from build123d import *

# Parameters (mm, degrees)
SKETCH1_R               = 1.75
BOSS_EXTRUDE1_DEPTH     = 1.5
BOSS_EXTRUDE2_START     = -72
BOSS_EXTRUDE2_DEPTH     = 72
BOSS_EXTRUDE4_DEPTH     = 2
SKETCH5_R               = 1.75
CUT_EXTRUDE1_DEPTH      = 2
CUT_EXTRUDE2_DEPTH      = 152.713437324
CUT_EXTRUDE2_DEPTH_BACK = 152.713437324
SKETCH6_W               = 72
SKETCH6_H               = 11.5
FILLET1_R               = 2
SKETCH8_W               = 36
SKETCH8_H               = 18
CUT_EXTRUDE3_DEPTH      = 22.4262221
SKETCH11_W              = 3
SKETCH11_H              = 15
BOSS_EXTRUDE7_DEPTH     = 15
CUT_EXTRUDE5_REACH      = 154.64
FILLET3_R               = 5


with BuildPart() as part:
    # Sketch1 → Boss-Extrude1 (new body)
    with BuildSketch(Plane.XY):
        with BuildLine():
            Line((-32.5, -138.9), (32.5, -138.9))
            Line((32.5, -138.9), (36, -138.9))
            Line((36, -138.9), (36, -136.815047169))
            ThreePointArc((36, -136.815047169), (37.65, -133.9), (36, -130.984952831))
            Line((36, -130.984952831), (36, -8.615047169))
            ThreePointArc((36, -8.615047169), (37.65, -5.7), (36, -2.784952831))
            Line((36, -2.784952831), (36, 0))
            Line((36, 0), (-36, 0))
            Line((-36, 0), (-36, -2.784952831))
            ThreePointArc((-36, -2.784952831), (-37.65, -5.7), (-36, -8.615047169))
            Line((-36, -8.615047169), (-36, -130.984952831))
            ThreePointArc((-36, -130.984952831), (-37.65, -133.9), (-36, -136.815047169))
            Line((-36, -136.815047169), (-36, -138.9))
            Line((-36, -138.9), (-32.5, -138.9))
        make_face()
        with Locations((-34.25, -133.9)):
            Circle(SKETCH1_R, mode=Mode.SUBTRACT)
        with Locations((34.25, -133.9)):
            Circle(SKETCH1_R, mode=Mode.SUBTRACT)
        with Locations((34.25, -5.7)):
            Circle(SKETCH1_R, mode=Mode.SUBTRACT)
        with Locations((-34.25, -5.7)):
            Circle(SKETCH1_R, mode=Mode.SUBTRACT)
    extrude(amount=BOSS_EXTRUDE1_DEPTH)

    # Sketch2 → Boss-Extrude2 (add)
    with BuildSketch(Plane.ZY.offset(36).offset(BOSS_EXTRUDE2_START)):
        Polygon((1.5, -141.1), (1.5, -138.9), (0, -138.9), (0, -139.1), (-40, -139.1), (-40, -141.1), align=None)
    extrude(amount=BOSS_EXTRUDE2_DEPTH)

    # Sketch4 → Boss-Extrude4 (add)
    with BuildSketch(Plane.XZ.offset(141.1)):
        with BuildLine():
            Line((-36, -15.904411924), (-36, -24.211404996))
            ThreePointArc((-36, -24.211404996), (-38.768391924, -20.05790846), (-36, -15.904411924))
        make_face()
        with BuildLine():
            Line((36, -15.879321263), (36, -24.236495657))
            ThreePointArc((36, -24.236495657), (38.8298476, -20.05790846), (36, -15.879321263))
        make_face()
    extrude(amount=-BOSS_EXTRUDE4_DEPTH)

    # Sketch5 → Cut-Extrude1 (cut)
    with BuildSketch(Plane.XZ.offset(141.1)):
        with Locations(Location((-34.25, -20, 0), (0, 0, 270))):
            Circle(SKETCH5_R)
        with Locations(Location((34.25, -20, 0), (0, 0, 270))):
            Circle(SKETCH5_R)
    extrude(amount=-CUT_EXTRUDE1_DEPTH, mode=Mode.SUBTRACT)

    # Sketch6 → Cut-Extrude2 (cut, two sides: drawn at the far end of the back side and taken through both)
    with BuildSketch(Plane.XZ.offset(141.1).offset(-CUT_EXTRUDE2_DEPTH_BACK)):
        with Locations((0, -34.25)):
            Rectangle(SKETCH6_W, SKETCH6_H)
    extrude(amount=CUT_EXTRUDE2_DEPTH + CUT_EXTRUDE2_DEPTH_BACK, mode=Mode.SUBTRACT)

    # Fillet1
    fillet1_edges = [part.edges().sort_by_distance(p)[0] for p in [
        (36, -140.1, -28.5),
        (-36, -140.1, -28.5),
    ]]
    fillet(fillet1_edges, radius=FILLET1_R)

    # Sketch8 → Cut-Extrude3 (cut)
    with BuildSketch(Plane.XZ.offset(141.1)):
        with Locations((-9, -14.5)):
            Rectangle(SKETCH8_W, SKETCH8_H)
    extrude(amount=-CUT_EXTRUDE3_DEPTH, mode=Mode.SUBTRACT)

    # Sketch11 → Boss-Extrude7 (add)
    with BuildSketch(Plane(origin=(0, -139.1, 0), x_dir=(1, 0, 0), z_dir=(0, 1, 0))):
        with Locations((10.5, 7.5)):
            Rectangle(SKETCH11_W, SKETCH11_H)
    extrude(amount=BOSS_EXTRUDE7_DEPTH)

    # Sketch12 → Cut-Extrude5 (cut, up to next)
    with BuildSketch(Plane(origin=(12, 0, 0), x_dir=(0, 0, -1), z_dir=(1, 0, 0)), mode=Mode.PRIVATE) as cut_extrude5_sk1:
        Polygon((0, -124.1), (15, -139.1), (15, -124.1), align=None)
    cut_extrude5_tool1 = extrude(cut_extrude5_sk1.sketch, amount=-CUT_EXTRUDE5_REACH, mode=Mode.PRIVATE) & part.part
    add(cut_extrude5_tool1.solids().sort_by_distance((12, -129.1, -10))[0], mode=Mode.SUBTRACT)

    # Fillet3
    fillet3_edges = [part.edges().sort_by_distance(p)[0] for p in [
        (36, -140.1, -24.236495657),
        (36, -140.1, -15.879321263),
        (-36, -140.1, -15.904411924),
        (-36, -140.1, -24.211404996),
    ]]
    fillet(fillet3_edges, radius=FILLET3_R)


solid = part.part
The listing builds one solid part. Answer for the finished solid, in the listing's coordinates (mm). A direction names the side the tool comes from. Round coordinates to 2 decimals unless told otherwise and drop trailing zeros. Write each loop counter-clockwise with the first axis right and the second up, starting at its lowest first coordinate (ties: lowest second). Pieces come first, ordered by that corner, then holes. Notation, with made-up numbers: (39.5, 50) - (55.5, 50) arc R22 cw to (55.5, 56) - close; hole circle Ø9 at (43.5, -12.5). An arc over 180 degrees is marked (long way). Use a Markdown table: item, result. Add a question column.
1. A tool of negligible diameter and unlimited length cuts with its end or side. For faces 1 (the face through (36, -140, -6)), 2 (the face through (9, -136, -6)), 3 (the face through (-36, -140, -6)), 4 (the face through (12, -133, -6)), from which of +Z, -Z, +X, -X, +Y, -Y can it reach the whole face along a straight path? Write none if from no direction.
2. Consider line 1 (Y direction, x = -34.25, z = 0.45); line 2 (X direction, y = -139.7, z = -20); line 3 (X direction, y = -133.9, z = 0.9). Determine where each line is inside the solid, lowest interval first.
3. Flat-ended cylindrical pins translate along their axes: P1, Ø7.5, axis at y = -131, z = -6, coming from the +X side; P2, Ø3.5, axis at y = -139.5, z = -7, coming from the -X side; P3, Ø4, axis at x = 28.5, y = -117, coming from the -Z side. Find the tip coordinate at first contact, or state that the pin passes through.
4. The part is cut by section B-B (x = -4). Write down the section's boundary in (y, z).
5. For a pull along Z with two mould halves and no side action, classify faces 5 (the face through (34.33, -140.11, -18.25)), 6 (the face through (10.5, -131.5, -7.4)), 7 (the face through (-34.63, -135.61, 0.74)), 8 (the face through (-34.17, -140.11, -18.25)) as +Z half, -Z half, draft (parallel to the pull), parting line (faces both ways), or undercut.
6. The part is cut by section A-A (z = -8.5). Write down the section's boundary in (x, y).
7. The part is cut by section D-D (z = -2.5). Write down the section's boundary in (x, y), and give its area (4 significant figures).
8. The part is cut by section C-C (y = -133.9). Write down the section's boundary in (x, z).
Reported:
| question | item | result |
|---|---|---|
| 1 | face 1 | +Z, +X, -Y |
| 1 | face 2 | +Y |
| 1 | face 3 | +Z, -X, -Y |
| 1 | face 4 | -Z, +X, +Y |
| 2 | line 1 | -141.1 to -135.65, -132.15 to -7.45, -3.95 to 0 |
| 2 | line 2 | -38.77 to -36, -32.5 to -27, 9 to 32.5, 36 to 38.83 |
| 2 | line 3 | -37.65 to -36, -32.5 to 32.5, 36 to 37.65 |
| 3 | P1 | x = 12 |
| 3 | P2 | x = -36 |
| 3 | P3 | z = 0 |
| 4 | outline | (-141.1, -28.5) - (-139.1, -28.5) - (-139.1, -23.5) - (-141.1, -23.5) - close; (-141.1, -5.5) - (-139.1, -5.5) - (-139.1, 0) - (0, 0) - (0, 1.5) - (-141.1, 1.5) - close |
| 5 | face 5 | undercut |
| 5 | face 6 | -Z half |
| 5 | face 7 | draft |
| 5 | face 8 | undercut |
| 6 | outline | (-36, -141.1) - (-27, -141.1) - (-27, -139.1) - (-36, -139.1) - close; (9, -141.1) - (36, -141.1) - (36, -139.1) - (12, -139.1) - (12, -132.6) - (9, -132.6) - close |
| 7 | outline | (-36, -141.1) - (36, -141.1) - (36, -139.1) - (12, -139.1) - (12, -126.6) - (9, -126.6) - (9, -139.1) - (-36, -139.1) - close |
| 7 | area | 181.5 mm^2 |
| 8 | outline | (-37.65, 0) - (-36, 0) - (-36, 1.5) - (-37.65, 1.5) - close; (-32.5, 0) - (9, 0) - (9, -9.8) - (12, -9.8) - (12, 0) - (32.5, 0) - (32.5, 1.5) - (-32.5, 1.5) - close; (36, 0) - (37.65, 0) - (37.65, 1.5) - (36, 1.5) - close |
